Geometry check sheet. Reference: the model listing, model coordinates, mm. Face numbers are marked on the shaded views. A direction names the side the tool comes from. Round coordinates to 2 decimals unless told otherwise and drop trailing zeros. Order: outer loops, then holes, each group sorted by start corner. A loop starts at its lowest first (then second) coordinate and runs counter-clockwise, first axis right, second up.
(1) Set-up check for the marked faces 4, 5 and 6: record each of +Z, -Z, +X, -X, +Y, -Y from which the full face is reachable in a straight line by a thin tool's end or side.
(2) Thickness scan on L1, parallel to Y at x = 0, z = 15; L2, parallel to Y at x = -39, z = 33.5; L3, parallel to Y at x = 11, z = 6.5. Record the ranges inside material, lowest first.
(3) Cross-section at C-C on z = 17. Enter the section's corners in (x, y).
(4) Cross-section at A-A on y = 0. Enter the section's corners in (x, z), and give its area (3 significant figures).
(5) Draft check along Y on the marked faces 1, 2 and 3. Enter one of: pulls with the +Y half, pulls with the -Y half, needs draft (parallel to the pull), parting line crosses it, or undercut.
(6) Gauge pin test, flat ends, axial feed: P1, Ø6.5, axis at x = 24, z = 30, coming from the +Y side; P2, Ø1.5, axis at x = -28, y = 24.5, coming from the -Z side; P3, Ø5, axis at x = 40.5, z = 15.5, coming from the -Y side. Record the tip position at first contact, or that the pin passes through.
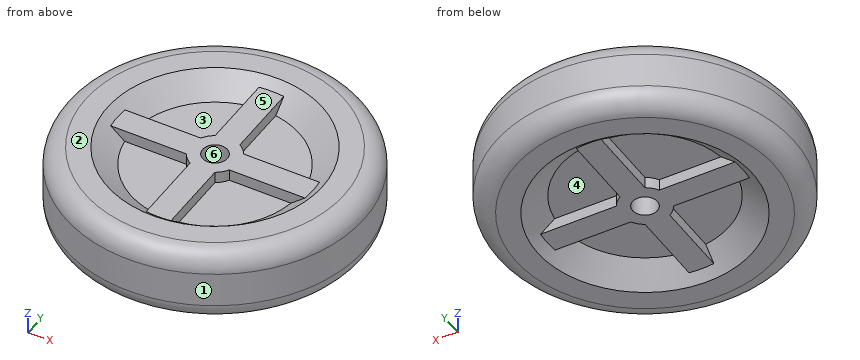
from build123d import *

# Parameters (mm, degrees)
SKETCH1_R               = 76.2
BOSS_EXTRUDE1_DEPTH     = 38.1
FILLET1_R               = 10
SKETCH2_R               = 6.35
CUT_EXTRUDE1_DEPTH      = 38.1
SKETCH3_R               = 55
CUT_EXTRUDE2_DEPTH      = 10
CUT_EXTRUDE2_DRAFT      = -50
MIRROR1_COPY_1_SKETCH_R = 55
MIRROR1_COPY_1_DEPTH    = 10
MIRROR1_COPY_1_DRAFT    = -50
SKETCH4_R               = 6.35
BOSS_EXTRUDE3_DEPTH     = 15


with BuildPart() as part:
    # Sketch1 → Boss-Extrude1 (new body)
    with BuildSketch(Plane.XY):
        with Locations(Location((0, 0, 0), (0, 0, 180))):
            Circle(SKETCH1_R)
    extrude(amount=BOSS_EXTRUDE1_DEPTH)

    # Fillet1
    fillet1_edges = [part.edges().sort_by_distance(p)[0] for p in [
        (76.2, 0, 0),
        (76.2, 0, 38.1),
    ]]
    fillet(fillet1_edges, radius=FILLET1_R)

    # Sketch2 → Cut-Extrude1 (cut)
    with BuildSketch(Plane.XY.offset(38.1)):
        Circle(SKETCH2_R)
    extrude(amount=-CUT_EXTRUDE1_DEPTH, mode=Mode.SUBTRACT)


with BuildPart() as cut_extrude2_tool:
    # Sketch3 → Cut-Extrude2 (with draft: the straight prism first)
    with BuildSketch(Plane.XY.offset(38.1)):
        Circle(SKETCH3_R)
    extrude(amount=-CUT_EXTRUDE2_DEPTH)
    # Cut-Extrude2: the draft: its side faces are tilted about the plane it starts from
    cut_extrude2_sides = [cut_extrude2_tool.faces().sort_by_distance(p)[0] for p in [
        (-55, 0, 33.1),
    ]]
    draft(cut_extrude2_sides, Plane.XY.offset(38.1), CUT_EXTRUDE2_DRAFT)


with BuildPart() as part_1:
    add(part.part)

    # Cut-Extrude2: cut by cut_extrude2_tool
    add(cut_extrude2_tool.part, mode=Mode.SUBTRACT)


with BuildPart() as mirror1_copy_1_tool:
    # Mirror1 copy 1 sketch → Mirror1 copy 1 (with draft: the straight prism first)
    with BuildSketch(Plane(origin=(0, 0, 0), x_dir=(1, 0, 0), z_dir=(0, 0, -1))):
        Circle(MIRROR1_COPY_1_SKETCH_R)
    extrude(amount=-MIRROR1_COPY_1_DEPTH)
    # Mirror1 copy 1: the draft: its side faces are tilted about the plane it starts from
    mirror1_copy_1_sides = [mirror1_copy_1_tool.faces().sort_by_distance(p)[0] for p in [
        (-55, 0, 5),
    ]]
    draft(mirror1_copy_1_sides, Plane(origin=(0, 0, 0), x_dir=(1, 0, 0), z_dir=(0, 0, -1)), MIRROR1_COPY_1_DRAFT)


with BuildPart() as part_2:
    add(part_1.part)

    # Mirror1 copy 1: cut by mirror1_copy_1_tool
    add(mirror1_copy_1_tool.part, mode=Mode.SUBTRACT)

    # Sketch4 → Boss-Extrude3 (add, symmetric)
    with BuildSketch(Plane(origin=(0, 0, 19.05), x_dir=(-1, 0, 0), z_dir=(0, 0, -1))):
        with BuildLine():
            Line((10.998522628, 6.35), (54.632202042, 6.35))
            Line((54.632202042, 6.35), (54.632202042, -6.35))
            Line((54.632202042, -6.35), (10.998522628, -6.35))
            ThreePointArc((10.998522628, -6.35), (8.980256121, -8.980256121), (6.35, -10.998522628))
            Line((6.35, -10.998522628), (6.35, -54.632202042))
            Line((6.35, -54.632202042), (-6.35, -54.632202042))
            Line((-6.35, -54.632202042), (-6.35, -10.998522628))
            ThreePointArc((-6.35, -10.998522628), (-8.980256121, -8.980256121), (-10.998522628, -6.35))
            Line((-10.998522628, -6.35), (-54.632202042, -6.35))
            Line((-54.632202042, -6.35), (-54.632202042, 6.35))
            Line((-54.632202042, 6.35), (-10.998522628, 6.35))
            ThreePointArc((-10.998522628, 6.35), (-8.980256121, 8.980256121), (-6.35, 10.998522628))
            Line((-6.35, 10.998522628), (-6.35, 54.632202042))
            Line((-6.35, 54.632202042), (6.35, 54.632202042))
            Line((6.35, 54.632202042), (6.35, 10.998522628))
            ThreePointArc((6.35, 10.998522628), (8.980256121, 8.980256121), (10.998522628, 6.35))
        make_face()
        with Locations(Location((0, 0, 0), (0, 0, 180))):
            Circle(SKETCH4_R, mode=Mode.SUBTRACT)
    extrude(amount=BOSS_EXTRUDE3_DEPTH, both=True)


solid = part_2.part
Found:
1. face 4: -Z
1. face 5: +Z
1. face 6: +Z, -Z
2. L1: y = -76.2 to -6.35, 6.35 to 76.2
2. L2: y = -63.61 to -30.51, -6.35 to 6.35, 30.51 to 63.61
2. L3: y = -74.76 to -45.96, -6.35 to 6.35, 45.96 to 74.76
3. outline: circle Ø152.4 at (0, 0); hole circle Ø12.7 at (0, 0)
4. outline: (-76.2, 10) arc R10 ccw to (-66.2, 0) - (-55, 0) - (-50.17, 4.05) - (-6.35, 4.05) - (-6.35, 34.05) - (-50.17, 34.05) - (-55, 38.1) - (-66.2, 38.1) arc R10 ccw to (-76.2, 28.1) - close; (6.35, 4.05) - (50.17, 4.05) - (55, 0) - (66.2, 0) arc R10 ccw to (76.2, 10) - (76.2, 28.1) arc R10 ccw to (66.2, 38.1) - (55, 38.1) - (50.17, 34.05) - (6.35, 34.05) - close
4. area: 4,490 mm2
5. face 1: parting line crosses it
5. face 2: needs draft
5. face 3: undercut
6. P1: stops at y = 73.23
6. P2: stops at z = 10
6. P3: stops at y = -66.05
